For this review, use the dimensioned drawing (mm, ordinates from the lowest corner) and the shaded views. A direction names the side the tool comes from. Round coordinates to 2 decimals unless told otherwise and drop trailing zeros. Loops run counter-clockwise (first coordinate to the right, second up) from the corner with the lowest first, then second, coordinate; pieces in that order, holes last. Notation, with made-up numbers: (-2, 43) - (12, 43) arc R20 ccw to (12, 69) - close; hole circle Ø7 at (-1.5, 24.5). An arc over 180 degrees is marked (long way). One line per question, with ' | ' between items. Start each with the question number.
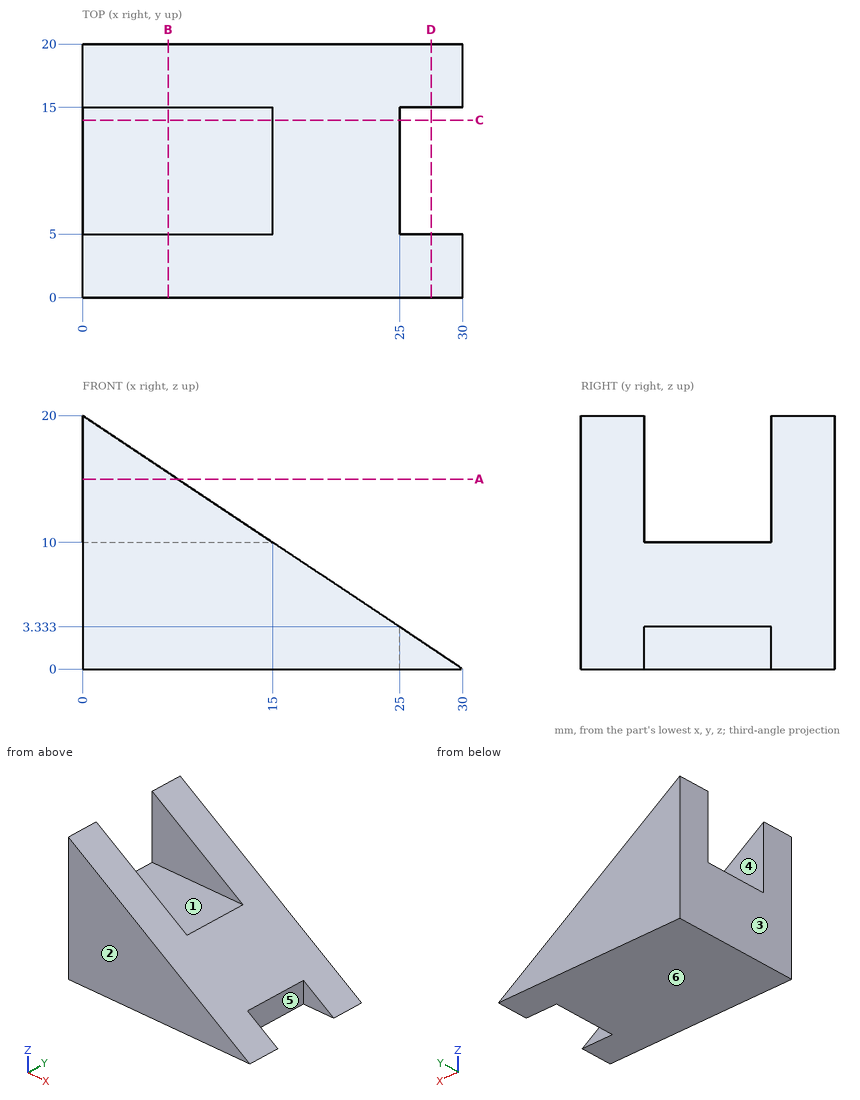
1. Machinability: for the marked faces 4, 5 and 6, which of the approach directions +Z, -Z, +X, -X, +Y, -Y give a long, thin tool a straight path to every point of the face, cutting with its end or side? Answer none if there is none.
2. Take a section at A-A, the plane z = 15. Give the boundary of the cut face in (x, y), then the cut area to 3 significant figures.
3. Take a section at B-B, the plane x = 6.75. Give the boundary of the cut face in (y, z), then the cut area to 3 significant figures.
4. To check wall thickness, follow line 1 along Z through (x, y) = (6.25, 6.25); line 2 along Z through (x, y) = (18, 17.25); line 3 along X through (y, z) = (16, 9.75) (1 decimal). State the ranges of each line that lie inside material, in increasing order.
5. Take a section at C-C, the plane y = 14. Give the boundary of the cut face in (x, z).
6. The part is to be moulded in two halves that separate along Y. For the marked faces 1, 2 and 3, say which applies: pulls with the +Y half, pulls with the -Y half, needs draft (parallel to the pull), parting line crosses it, or undercut.
7. Take a section at D-D, the plane x = 27.5. Give the boundary of the cut face in (y, z).
8. Clearance check with flat-ended pins moving along their axes: P1, Ø5, axis at x = 23.5, y = 17.5, coming from the -Z side; P2, Ø3, axis at x = 8, z = 17.5, coming from the +Y side; P3, Ø8, axis at x = 4.5, y = 10, coming from the +Z side; P4, Ø1.7, axis at y = 10.5, z = 2.5, coming from the +X side. State where each tip first meets the part, or that it passes through.
Answer list:
1) face 4: +Z, +X, -X | face 5: +Z, -Z, +X | face 6: -Z, +X, -X, +Y, -Y
2) outline: (0, 0) - (7.5, 0) - (7.5, 5) - (0, 5) - close; (0, 15) - (7.5, 15) - (7.5, 20) - (0, 20) - close | area: 75.0 mm²
3) outline: (0, 0) - (20, 0) - (20, 15.5) - (15, 15.5) - (15, 10) - (5, 10) - (5, 15.5) - (0, 15.5) - close | area: 255 mm²
4) line 1: z = 0 to 10 | line 2: z = 0 to 8 | line 3: x = 0 to 15.4
5) outline: (0, 0) - (25, 0) - (25, 3.33) - (15, 10) - (0, 10) - close
6) face 1: undercut | face 2: pulls with the -Y half | face 3: needs draft
7) outline: (0, 0) - (5, 0) - (5, 1.67) - (0, 1.67) - close; (15, 0) - (20, 0) - (20, 1.67) - (15, 1.67) - close
8) P1: stops at z = 0 | P2: passes through | P3: stops at z = 10 | P4: stops at x = 25
